Part model, mm, in its own coordinate system. Face numbers are marked on the shaded views. Round coordinates to 2 decimals unless told otherwise and drop trailing zeros. Loops run counter-clockwise (first coordinate to the right, second up) from the corner with the lowest first, then second, coordinate; pieces in that order, holes last. Notation, with made-up numbers: M -33.5,40.5 L 6.5,40.5 A19 ccw 6.5,74.5 Z; hole C 49,-16 d5. An arc over 180 degrees is marked long. Put each result on its own line as item: value. Start each with the question number.
1) Slice it at D-D on z = 71. Give the cut face in (x, y).
2) Slice it at B-B on y = 0. Give the cut face in (x, z), then the cut area to 3 significant figures.
3) Slice it at C-C on x = 0. Give the cut face in (y, z).
4) Slice it at A-A on x = -10.5. Give the cut face in (y, z).
5) Probe line 1 along Y through (x, z) = (0, 7); line 2 along Z through (x, y) = (-23, 14.5); line 3 along Z through (x, y) = (19, 32). List the from-to ranges inside material, lowest first.
6) Pull direction Y, two halves, no side cores. Call the marked faces 1, 2 and 3: +Y half, -Y half, draft (parallel to the pull), parting line (faces both ways), or undercut.
7) Drop flat-ended pins along their axis: pin 1 Ø1.8 at (y, z) = (30.5, 36) entering from +X; pin 2 Ø4 at (x, y) = (-19.5, 31) entering from +Z; pin 3 Ø3 at (x, y) = (28.5, -21.5) entering from -Z; pin 4 Ø3 at (y, z) = (31.5, 77) entering from +X. Give the stop position or say it passes through.
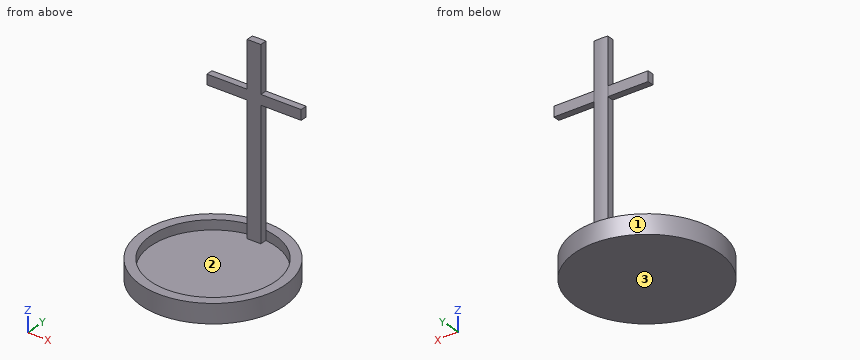
```python
from build123d import *

# Parameters (mm, degrees)
F0_R     = 38.1
F1_DEPTH = 10.16
F2_T     = -5.08
F4_DEPTH = 98.552
F5_W     = 3.5759293783
F5_H     = 5.342617631
F6_DEPTH = 25.146


with BuildPart() as f1:
    # F0 (on Top) → F1 (new body)
    with BuildSketch(Plane.XY):
        Circle(F0_R)
    extrude(amount=F1_DEPTH)

    # F2
    f2_openings = [f1.faces().sort_by_distance(p)[0] for p in [
        (0, 0, 10.16),
    ]]
    offset(amount=F2_T, openings=f2_openings)

    # F3 (on face) → F4 (join)
    with BuildSketch(Plane.XY.offset(5.08)):
        with BuildLine():
            Line((-3.6385965068, 29.2429830879), (3.6385965068, 29.2429830879))
            Line((3.6385965068, 29.2429830879), (3.6385965068, 32.8189124661))
            ThreePointArc((3.6385965068, 32.8189124661), (0, 33.02), (-3.6385965068, 32.8189124661))
            Line((-3.6385965068, 32.8189124661), (-3.6385965068, 29.2429830879))
        make_face()
    extrude(amount=F4_DEPTH)

    # F5 (on Right) → F6 (join, symmetric)
    with BuildSketch(Plane.YZ):
        with Locations((31.030947777, 76.2954577804)):
            Rectangle(F5_W, F5_H)
    extrude(amount=F6_DEPTH, both=True)


solid = f1.part
```
Recorded:
1. outline: M -3.64,29.24 L 3.64,29.24 L 3.64,32.82 A33.02 ccw -3.64,32.82 Z
2. outline: M -38.1,0 L 38.1,0 L 38.1,10.16 L 33.02,10.16 L 33.02,5.08 L -33.02,5.08 L -33.02,10.16 L -38.1,10.16 Z
2. area: 439 mm2
3. outline: M -38.1,0 L 38.1,0 L 38.1,10.16 L 33.02,10.16 L 33.02,103.63 L 29.24,103.63 L 29.24,5.08 L -33.02,5.08 L -33.02,10.16 L -38.1,10.16 Z
4. outline: M -36.62,0 L 36.62,0 L 36.62,10.16 L 31.31,10.16 L 31.31,5.08 L -31.31,5.08 L -31.31,10.16 L -36.62,10.16 Z; M 29.24,73.62 L 32.82,73.62 L 32.82,78.97 L 29.24,78.97 Z
5. line 1: y = -38.1 to -33.02, 29.24 to 38.1
5. line 2: z = 0 to 5.08
5. line 3: z = 0 to 10.16, 73.62 to 78.97
6. face 1: parting line
6. face 2: undercut
6. face 3: draft
7. pin 1: stops at x = 3.64
7. pin 2: stops at z = 78.97
7. pin 3: stops at z = 0
7. pin 4: stops at x = 25.15
